```python
from build123d import *

# Parameters (mm, degrees)
SKETCH1_W        = 38.1
SKETCH1_H        = 482.6
EXTRUSION1_DEPTH = 3.175
HOLE1_D          = 6.35
HOLE2_D          = 12.7
EXTRUSION2_START = -3.175
SKETCH6_R        = 6.35
EXTRUSION2_DEPTH = 3.175
HOLE3_D          = 12.7
HOLE4_D          = 3.96875


with BuildPart() as part:
    # Sketch1 → Extrusion1 (new body)
    with BuildSketch(Plane(origin=(0, 0, 0), x_dir=(-1, 0, 0), z_dir=(0, 1, 0))):
        Rectangle(SKETCH1_W, SKETCH1_H)
    extrude(amount=EXTRUSION1_DEPTH)

    # Hole1 (through all)
    with Locations(Plane(origin=(0, 3.175, 0), x_dir=(1, 0, 0), z_dir=(0, 1, 0))):
        with Locations((0, -228.6), (0, 228.6), (0, 0)):
            Hole(HOLE1_D / 2)

    # Hole2 (through all)
    with Locations(Plane(origin=(0, 3.175, 0), x_dir=(1, 0, 0), z_dir=(0, 1, 0))):
        with Locations((0, -101.6), (0, 101.6)):
            Hole(HOLE2_D / 2)

    # Sketch6 → Extrusion2 (add)
    with BuildSketch(Plane(origin=(0, 3.175, 0), x_dir=(1, 0, 0), z_dir=(0, 1, 0)).offset(EXTRUSION2_START)):
        with Locations((0, -101.6)):
            Circle(SKETCH6_R)
        with Locations((0, 101.6)):
            Circle(SKETCH6_R)
    extrude(amount=EXTRUSION2_DEPTH)

    # Hole3 (through all)
    with Locations(Plane(origin=(0, 3.175, 0), x_dir=(1, 0, 0), z_dir=(0, 1, 0))):
        with Locations((0, 114.3), (0, -114.3)):
            Hole(HOLE3_D / 2)

    # Hole4 (through all)
    with Locations(Plane(origin=(0, 3.175, 0), x_dir=(1, 0, 0), z_dir=(0, 1, 0))):
        with Locations((0, -88.9), (0, -139.7), (0, 88.9), (0, 139.7)):
            Hole(HOLE4_D / 2)


solid = part.part
```
Part model, mm, in its own coordinate system. Round coordinates to 2 decimals unless told otherwise and drop trailing zeros. Write each loop counter-clockwise with the first axis right and the second up, starting at its lowest first coordinate (ties: lowest second). Pieces come first, ordered by that corner, then holes. Notation, with made-up numbers: (53, -23) -> (71, -23) arc R23 ccw to (71, 13) -> close; hole circle Ø11 at (23.25, 78). An arc over 180 degrees is marked (long way). Return JSON: item names as keys, results as strings. Group by question number.
Q1. Mould opens along Z. For faces 1 (the cylindrical face through (1.38, 1.57, -108.1)), 2 (the flat face through (0.3, 3.175, 3.4)) say: pulls with the +Z half, pulls with the -Z half, needs draft (parallel to the pull), parting line crosses it, or undercut.
Q2. Probe L1, parallel to Z at x = 4, y = 2.4; L2, parallel to X at y = 1.05, z = 228.6 (3 decimals); L3, parallel to X at y = 1.45, z = 88.9. List the from-to ranges inside material, lowest first. Write a range as [from, to].
Q3. Pin check, flat tips, straight feed: pin 1 (5 mm diameter, centred on x = 0, z = -139.7, fed in from +Y) (3 decimals); pin 2 (4 mm diameter, centred on x = 0, z = 0, fed in from +Y). Stop position of each tip, or through.
Q4. Saw through at B-B on y = 2.55. State how many separate pieces and enclosed holes the cut face has, plus the area to 3 significant figures.
Q5. Saw through at A-A on z = -114.3. Write the cut outline in (x, y) (3 decimals).
Answer:
{
 "1": {"face 1": "undercut", "face 2": "needs draft"},
 "2": {"L1": "[-241.3, -119.23], [-109.37, 109.37], [119.23, 241.3]", "L2": "[-19.05, -3.175], [3.175, 19.05]", "L3": "[-19.05, -1.98], [1.98, 19.05]"},
 "3": {"pin 1": "y = 3.175", "pin 2": "through"},
 "4": {"separate pieces": "1", "enclosed holes": "9", "area": "18,000 mm2"},
 "5": {"outline": "(-19.05, 0) -> (-6.35, 0) -> (-6.35, 3.175) -> (-19.05, 3.175) -> close; (6.35, 0) -> (19.05, 0) -> (19.05, 3.175) -> (6.35, 3.175) -> close"}
}
